from build123d import *

# Parameters (mm, degrees)
EXTRUDE_1_DEPTH       = 245
EXTRUDE_3_DEPTH       = 245
PATTERN_CURVE_1_COUNT = 19
PATTERN_CURVE_1_PITCH = 9.75
SKETCH_3_R            = 2.05
CUT_EXTRUDE_1_DEPTH   = 10
CUT_EXTRUDE_START     = -10
SKETCH_5_R            = 2.05
CUT_EXTRUDE_2_DEPTH   = 10
SKETCH_6_R            = 2.5
CUT_EXTRUDE_3_DEPTH   = 8
SKETCH_7_R            = 2.6
CUT_EXTRUDE_4_DEPTH   = 6
SKETCH_8_R            = 4.5
SKETCH_8_R_2          = 3.4
CUT_EXTRUDE_5_DEPTH   = 6
CUT_EXTRUDE_START_2   = -6
SKETCH_9_R            = 2.6
CUT_EXTRUDE_6_DEPTH   = 6
SKETCH_10_R           = 3.4
SKETCH_10_R_2         = 4.5
CUT_EXTRUDE_7_DEPTH   = 6
EXTRUDE_4_REACH       = 321.453
SKETCH_11_R           = 2.6
EXTRUDE_5_REACH       = 321.453
SKETCH_12_R           = 4.5
SKETCH_12_R_2         = 3.4
CUT_EXTRUDE_START_3   = -8
SKETCH_14_R           = 2.5
CUT_EXTRUDE_9_DEPTH   = 8
SKETCH_18_R           = 2.1
SKETCH_18_R_2         = 1.6
SKETCH_18_R_3         = 1.3
SKETCH_18_R_4         = 2.6
CUT_EXTRUDE_11_DEPTH  = 8


with BuildPart() as part:
    # Эскиз1 → Вытянуть1 (new body)
    with BuildSketch(Plane.XY):
        with BuildLine():
            Line((0, 45), (2.564446908, 45))
            ThreePointArc((2.564446908, 45), (3.247630994, 44.730246195), (3.562232066, 44.066519011))
            Line((3.562232066, 44.066519011), (5.5, 15))
            Line((5.5, 15), (194.5, 15))
            Line((194.5, 15), (196.437767934, 44.066519011))
            ThreePointArc((196.437767934, 44.066519011), (196.752369006, 44.730246195), (197.435553092, 45))
            Line((197.435553092, 45), (200, 45))
            Line((200, 45), (200, 0))
            Line((200, 0), (0, 0))
            Line((0, 0), (0, 45))
        make_face()
    extrude(amount=EXTRUDE_1_DEPTH)

    # Эскиз2 → Вытянуть3 (add)
    with BuildSketch(Plane.XY.offset(245)):
        with BuildLine():
            Line((11.5, 44.5), (10, 15))
            Line((10, 15), (14, 15))
            Line((14, 15), (12.5, 44.5))
            ThreePointArc((12.5, 44.5), (12, 45), (11.5, 44.5))
        make_face()
    extrude_3 = extrude(amount=-EXTRUDE_3_DEPTH)

    # Кривая1: Вытянуть3 ×19
    with Locations(*[(i * PATTERN_CURVE_1_PITCH, 0, 0) for i in range(1, PATTERN_CURVE_1_COUNT)]):
        add(extrude_3)

    # Эскиз3 → Вырез-Вытянуть1 (cut)
    with BuildSketch(Plane.XY.offset(245)):
        with Locations((20, 5)):
            Circle(SKETCH_3_R)
        with Locations((100, 5)):
            Circle(SKETCH_3_R)
        with Locations((180, 5)):
            Circle(SKETCH_3_R)
    extrude(amount=-CUT_EXTRUDE_1_DEPTH, mode=Mode.SUBTRACT)

    # Эскиз5 → Вырез-Вытянуть2 (cut)
    with BuildSketch(Plane(origin=(0, 0, 0), x_dir=(-1, 0, 0), z_dir=(0, 0, -1)).offset(CUT_EXTRUDE_START)):
        with Locations(Location((-180, 5, 0), (0, 0, 180))):
            Circle(SKETCH_5_R)
        with Locations(Location((-100, 5, 0), (0, 0, 180))):
            Circle(SKETCH_5_R)
        with Locations(Location((-20, 5, 0), (0, 0, 180))):
            Circle(SKETCH_5_R)
    extrude(amount=CUT_EXTRUDE_2_DEPTH, mode=Mode.SUBTRACT)

    # Эскиз6 → Вырез-Вытянуть3 (cut)
    with BuildSketch(Plane(origin=(0, 0, 0), x_dir=(-1, 0, 0), z_dir=(0, 0, -1))):
        with Locations((-4, 6)):
            Circle(SKETCH_6_R)
        with Locations(Location((-196, 6, 0), (0, 0, 180))):
            Circle(SKETCH_6_R)
    extrude(amount=-CUT_EXTRUDE_3_DEPTH, mode=Mode.SUBTRACT)

    # Эскиз7 → Вырез-Вытянуть4 (cut)
    with BuildSketch(Plane.ZY):
        with Locations(Location((22.5, 20, 0), (0, 0, 270))):
            Circle(SKETCH_7_R)
        with Locations(Location((222.5, 20, 0), (0, 0, 270))):
            Circle(SKETCH_7_R)
        with Locations(Location((122.5, 20, 0), (0, 0, 270))):
            Circle(SKETCH_7_R)
    extrude(amount=-CUT_EXTRUDE_4_DEPTH, mode=Mode.SUBTRACT)

    # Эскиз8 → Вырез-Вытянуть5 (cut)
    with BuildSketch(Plane(origin=(200, 0, 0), x_dir=(0, 0, -1), z_dir=(1, 0, 0))):
        with Locations((-80, 30)):
            Circle(SKETCH_8_R)
        with Locations((-165, 30)):
            Circle(SKETCH_8_R_2)
    extrude(amount=-CUT_EXTRUDE_5_DEPTH, mode=Mode.SUBTRACT)

    # Эскиз9 → Вырез-Вытянуть6 (cut)
    with BuildSketch(Plane(origin=(200, 0, 0), x_dir=(0, 0, -1), z_dir=(1, 0, 0)).offset(CUT_EXTRUDE_START_2)):
        with Locations(Location((-22.5, 20, 0), (0, 0, 270))):
            Circle(SKETCH_9_R)
        with Locations(Location((-122.5, 20, 0), (0, 0, 270))):
            Circle(SKETCH_9_R)
        with Locations(Location((-222.5, 20, 0), (0, 0, 270))):
            Circle(SKETCH_9_R)
    extrude(amount=CUT_EXTRUDE_6_DEPTH, mode=Mode.SUBTRACT)

    # Эскиз10 → Вырез-Вытянуть7 (cut)
    with BuildSketch(Plane.ZY.offset(CUT_EXTRUDE_START_2)):
        with Locations(Location((165, 30, 0), (0, 0, 180))):
            Circle(SKETCH_10_R)
        with Locations(Location((80, 30, 0), (0, 0, 180))):
            Circle(SKETCH_10_R_2)
    extrude(amount=CUT_EXTRUDE_7_DEPTH, mode=Mode.SUBTRACT)

    # Вытянуть4: up to this face of the body (flat: up to its plane)
    extrude_4_end = Plane(part.part.faces().sort_by_distance((4.525743195, 29.613852069, 122.666761542))[0])
    # Эскиз11 → Вытянуть4 (add, up to the picked face)
    with BuildSketch(Plane.ZY, mode=Mode.PRIVATE) as extrude_4_sk1:
        with Locations(Location((22.5, 20, 0), (0, 0, 180))):
            Circle(SKETCH_11_R)
    extrude_4_tool1 = split(extrude(extrude_4_sk1.sketch, amount=-EXTRUDE_4_REACH, mode=Mode.PRIVATE), bisect_by=extrude_4_end, keep=Keep.BOTH, mode=Mode.PRIVATE)
    # Эскиз11 → Вытянуть4 (add, up to the picked face)
    with BuildSketch(Plane.ZY, mode=Mode.PRIVATE) as extrude_4_sk2:
        with Locations(Location((122.5, 20, 0), (0, 0, 180))):
            Circle(SKETCH_11_R)
    extrude_4_tool2 = split(extrude(extrude_4_sk2.sketch, amount=-EXTRUDE_4_REACH, mode=Mode.PRIVATE), bisect_by=extrude_4_end, keep=Keep.BOTH, mode=Mode.PRIVATE)
    # Эскиз11 → Вытянуть4 (add, up to the picked face)
    with BuildSketch(Plane.ZY, mode=Mode.PRIVATE) as extrude_4_sk3:
        with Locations(Location((222.5, 20, 0), (0, 0, 180))):
            Circle(SKETCH_11_R)
    extrude_4_tool3 = split(extrude(extrude_4_sk3.sketch, amount=-EXTRUDE_4_REACH, mode=Mode.PRIVATE), bisect_by=extrude_4_end, keep=Keep.BOTH, mode=Mode.PRIVATE)
    add(extrude_4_tool1.solids().sort_by(Axis((0, 20, 22.5), (1, 0, 0)))[0])
    add(extrude_4_tool2.solids().sort_by(Axis((0, 20, 122.5), (1, 0, 0)))[0])
    add(extrude_4_tool3.solids().sort_by(Axis((0, 20, 222.5), (1, 0, 0)))[0])

    # Вытянуть5: up to this face of the body (flat: up to its plane)
    extrude_5_end = Plane(part.part.faces().sort_by_distance((195.474256805, 29.613852069, 122.666761542))[0])
    # Эскиз12 → Вытянуть5 (add, up to the picked face)
    with BuildSketch(Plane(origin=(200, 0, 0), x_dir=(0, 0, -1), z_dir=(1, 0, 0)), mode=Mode.PRIVATE) as extrude_5_sk1:
        with Locations(Location((-80, 30, 0), (0, 0, 270))):
            Circle(SKETCH_12_R)
    extrude_5_tool1 = split(extrude(extrude_5_sk1.sketch, amount=-EXTRUDE_5_REACH, mode=Mode.PRIVATE), bisect_by=extrude_5_end, keep=Keep.BOTH, mode=Mode.PRIVATE)
    # Эскиз12 → Вытянуть5 (add, up to the picked face)
    with BuildSketch(Plane(origin=(200, 0, 0), x_dir=(0, 0, -1), z_dir=(1, 0, 0)), mode=Mode.PRIVATE) as extrude_5_sk2:
        with Locations(Location((-165, 30, 0), (0, 0, 270))):
            Circle(SKETCH_12_R_2)
    extrude_5_tool2 = split(extrude(extrude_5_sk2.sketch, amount=-EXTRUDE_5_REACH, mode=Mode.PRIVATE), bisect_by=extrude_5_end, keep=Keep.BOTH, mode=Mode.PRIVATE)
    add(extrude_5_tool1.solids().sort_by(Axis((200, 30, 80), (-1, 0, 0)))[0])
    add(extrude_5_tool2.solids().sort_by(Axis((200, 30, 165), (-1, 0, 0)))[0])

    # Эскиз14 → Вырез-Вытянуть9 (cut)
    with BuildSketch(Plane.XY.offset(245).offset(CUT_EXTRUDE_START_3)):
        with Locations(Location((4, 6, 0), (0, 0, 180))):
            Circle(SKETCH_14_R)
        with Locations((196, 6)):
            Circle(SKETCH_14_R)
    extrude(amount=CUT_EXTRUDE_9_DEPTH, mode=Mode.SUBTRACT)

    # Эскиз18 → Вырез-Вытянуть11 (cut)
    with BuildSketch(Plane.XZ):
        with Locations((118, 203)):
            Circle(SKETCH_18_R)
        with Locations((63, 12.5)):
            Circle(SKETCH_18_R_2)
        with Locations((173, 12.5)):
            Circle(SKETCH_18_R_2)
        with Locations((173, 162.5)):
            Circle(SKETCH_18_R_2)
        with Locations((63, 162.5)):
            Circle(SKETCH_18_R_2)
        with Locations((101.5, 132.5)):
            Circle(SKETCH_18_R_3)
        with Locations((135, 132.5)):
            Circle(SKETCH_18_R_3)
        with Locations((148, 94.5)):
            Circle(SKETCH_18_R_4)
    extrude(amount=-CUT_EXTRUDE_11_DEPTH, mode=Mode.SUBTRACT)


solid = part.part
CAD build for the part. Positions are in the model's coordinates, mm. Coordinates: 2 decimals unless noted, no trailing zeros.
Item 1: Drill centre lines: L1, parallel to Y at x = 134, z = 205; L2, parallel to Z at x = 101, y = 6; L3, parallel to X at y = 6, z = 162. Where is each one in solid material? Low to high.
Check sheet entries:
L1: y = 0 to 15
L2: z = 10 to 131.3, 133.7 to 235
L3: x = 0 to 61.48, 64.52 to 171.48, 174.52 to 200
Item 2: Band-saw the part on A-A on y = 38.5. Give the number of separate pieces and of enclosed holes in the cut face, plus the area to 3 significant figures.
Check sheet entries:
separate pieces: 21
enclosed holes: 0
area: 9,420 mm2
Item 3: Pin check, flat tips, straight feed: pin 1 Ø3.5 at (x, y) = (20, 5) entering from -Z; pin 2 Ø4.5 at (x, z) = (95, 106.5) entering from +Y. Stop position of each tip, or through.
Check sheet entries:
pin 1: stops at z = 10
pin 2: stops at y = 15
Item 4: Two-plate mould, pull along Y, no slides. Class faces 1 (the face through (173, 15, 121)), 2 (the face through (101, 0, 121)), 3 (the face through (1.615, 6.751, 3.944)): +Y half, -Y half, draft (parallel to the pull), parting line (faces both ways), or undercut.
Check sheet entries:
face 1: +Y half
face 2: -Y half
face 3: undercut
